Check sheet for the modelled part. Datum: model origin and axes. Units: mm. Face numbers are marked on the shaded views. A direction names the side the tool comes from. Give positions to 0.01 mm unless a question says otherwise; leave off trailing zeros. Order: outer loops, then holes, each group sorted by start corner. A loop starts at its lowest first (then second) coordinate and runs counter-clockwise, first axis right, second up.
Item 1: Release check for a two-part mould opening along X. For the marked faces 1, 2 and 3 record: released by +X, released by -X, zero draft, split by the parting line, or undercut.
Item 2: Sectioned sample at A-A on x = -8.5. Record the boundary of the cut face in (y, z) (1 decimal), and give its area (3 significant figures).
Item 3: Access from +Z, -Z, +X, -X, +Y, -Y to the whole of each face (thin tool, end or side, straight path). Record for the marked faces 4 and 5.
Item 4: Material ranges on line 1 along X through (y, z) = (-4.75, 28.5), recorded low to high.
Item 5: Sectioned sample at C-C on z = 45.5. Record the boundary of the cut face in (x, y), and give its area (3 significant figures).
Item 6: Gauge pin test, flat end, axial feed: P1, Ø5, axis at x = 0.5, y = 8.5, coming from the +Z side. Record the tip position at first contact, or that the pin passes through.
from build123d import *

# Parameters (mm, degrees)
F1_W     = 25.4
F1_H     = 25.4
F2_DEPTH = 73.025
F3_T     = -1.5875
F4_DEPTH = 1.5885


# Not quite as in the source:
# - a variable given as a bare number and used for a length is read in inches; the dataset says mm whatever the document's units were


with BuildPart() as f2:
    # F1 (on Top) → F2 (new body)
    with BuildSketch(Plane.XY):
        Rectangle(F1_W, F1_H)
    extrude(amount=F2_DEPTH)

    # F3
    f3_openings = [f2.faces().sort_by_distance(p)[0] for p in [
        (0, 0, 73.025),
    ]]
    offset(amount=F3_T, openings=f3_openings)

    # F4 (cut, through all): a face of the model
    f4_faces = [f2.faces().sort_by_distance(p)[0] for p in [
        (0, 0, 1.5875),
    ]]
    extrude(f4_faces, amount=-F4_DEPTH, mode=Mode.SUBTRACT)


solid = f2.part
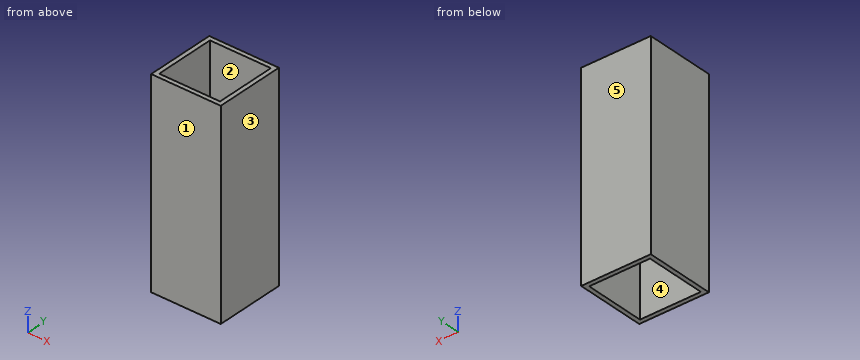
Report:
1. face 1: zero draft
1. face 2: undercut
1. face 3: released by +X
2. outline: (-12.7, 0) - (-11.1, 0) - (-11.1, 73) - (-12.7, 73) - close; (11.1, 0) - (12.7, 0) - (12.7, 73) - (11.1, 73) - close
2. area: 232 mm2
3. face 4: +Z, -Z
3. face 5: +Z, -Z, +X, -X, +Y
4. line 1: x = -12.7 to -11.11, 11.11 to 12.7
5. outline: (-12.7, -12.7) - (12.7, -12.7) - (12.7, 12.7) - (-12.7, 12.7) - close; hole (-11.11, -11.11) - (11.11, -11.11) - (11.11, 11.11) - (-11.11, 11.11) - close
5. area: 151 mm2
6. P1: passes through
